Geometry: final body of the model. Coordinates: model frame, mm. A direction names the side the tool comes from. Give positions to 0.01 mm unless a question says otherwise; leave off trailing zeros. Loops run counter-clockwise (first coordinate to the right, second up) from the corner with the lowest first, then second, coordinate; pieces in that order, holes last.
from build123d import *

# Parameters (mm, degrees)
BOSS_EXTRUDE1_DEPTH       = 34.31697226
SKETCH4_R                 = 19.05
BOSS_EXTRUDE2_DEPTH       = 12.7
SKETCH6_R                 = 12.7
BOSS_EXTRUDE3_DEPTH       = 88.9
SKETCH7_R                 = 6.35
CUT_EXTRUDE1_DEPTH        = 141.870111622
FILLET1_R                 = 5.08
FILLET2_R                 = 2.54
M6X1_0_TAPPED_HOLE1_D     = 5
M6X1_0_TAPPED_HOLE1_DEPTH = 41.148
M6X1_0_TAPPED_HOLE1_TIP   = 1.502151548


with BuildPart() as part:
    # Sketch3 → Boss-Extrude1 (new body)
    with BuildSketch(Plane(origin=(0, 0, 0), x_dir=(1, 0, 0), z_dir=(0, 1, 0))):
        Polygon((12.7, 0), (12.7, 12.7), (0, 12.7), (-12.7, 12.7), (-12.7, 0), (-12.7, -12.7), (0, -12.7), (12.7, -12.7), align=None)
    extrude(amount=BOSS_EXTRUDE1_DEPTH)

    # Sketch4 → Boss-Extrude2 (add)
    with BuildSketch(Plane(origin=(0, 34.31697226, 0), x_dir=(1, 0, 0), z_dir=(0, 1, 0))):
        with Locations(Location((0, 0, 0), (0, 0, 270))):
            Circle(SKETCH4_R)
    extrude(amount=BOSS_EXTRUDE2_DEPTH)

    # Sketch6 → Boss-Extrude3 (add)
    with BuildSketch(Plane(origin=(0, 47.01697226, 0), x_dir=(1, 0, 0), z_dir=(0, 1, 0))):
        with Locations(Location((0, 0, 0), (0, 0, 270))):
            Circle(SKETCH6_R)
    extrude(amount=BOSS_EXTRUDE3_DEPTH)

    # Sketch7 → Cut-Extrude1 (cut, through all)
    with BuildSketch(Plane.XY.offset(12.7)):
        with Locations((0, 12.7)):
            Circle(SKETCH7_R)
    extrude(amount=-CUT_EXTRUDE1_DEPTH, mode=Mode.SUBTRACT)

    # Fillet1
    fillet1_edges = [part.edges().sort_by_distance(p)[0] for p in [
        (12.7, 0, 0),
        (-12.7, 0, 0),
    ]]
    fillet(fillet1_edges, radius=FILLET1_R)

    # Fillet2
    fillet2_edges = [part.edges().sort_by_distance(p)[0] for p in [
        (0, 47.01697226, -12.7),
    ]]
    fillet(fillet2_edges, radius=FILLET2_R)

    # M6x1.0 Tapped Hole1
    with Locations(Plane(origin=(0, 135.91697226, 0), x_dir=(1, 0, 0), z_dir=(0, 1, 0))):
        with Locations((0, 0)):
            Hole(M6X1_0_TAPPED_HOLE1_D / 2, depth=M6X1_0_TAPPED_HOLE1_DEPTH)
            with Locations((0, 0, -(M6X1_0_TAPPED_HOLE1_DEPTH + M6X1_0_TAPPED_HOLE1_TIP / 2))):  # 118° drill point
                Cone(0, M6X1_0_TAPPED_HOLE1_D / 2, M6X1_0_TAPPED_HOLE1_TIP, mode=Mode.SUBTRACT)


solid = part.part
Item 1: Pin query (flat end, axial travel): pin 1 (5 mm diameter, centred on y = 53, z = 4.5, fed in from -X); pin 2 (20.5 mm diameter, centred on y = 20.5, z = -4, fed in from -X); pin 3 (3 mm diameter, centred on x = -9.5, z = -14.5, fed in from +Y). Return the tip coordinate at first contact, or that it passes through.
Values follow:
pin 1: stops at x = -12.54
pin 2: stops at x = -12.7
pin 3: stops at y = 47.02
Item 2: Section query D-D on y = 39. Return loops of the section in (x, z).
Values follow:
outline: circle Ø38.1 at (0, 0)
Item 3: Section query A-A on y = 12.7. Return loops of the section in (x, z).
Values follow:
outline: (-12.7, -12.7) - (-6.35, -12.7) - (-6.35, 12.7) - (-12.7, 12.7) - close; (6.35, -12.7) - (12.7, -12.7) - (12.7, 12.7) - (6.35, 12.7) - close
Item 4: Section query C-C on y = 85.5. Return loops of the section in (x, z), plus the area to 3 significant figures.
Values follow:
outline: circle Ø25.4 at (0, 0)
area: 507 mm2
Item 5: Section query B-B on y = 115.5. Return loops of the section in (x, z), plus the area to 3 significant figures.
Values follow:
outline: circle Ø25.4 at (0, 0); hole circle Ø5 at (0, 0)
area: 487 mm2
Item 6: Ray query, probe 1 along Y at (x, z) = (-3.5, -16); probe 2 along Z at (x, y) = (11, 28); probe 3 along Z at (x, y) = (-11, 67.5). Return the intervals inside material, ascending.
Values follow:
probe 1: y = 34.32 to 47.02
probe 2: z = -12.7 to 12.7
probe 3: z = -6.35 to 6.35
Item 7: Set-up query: faces 4 (the face through (0, 21, -12.7)), 5 (the face through (0, 21, 12.7)), 6 (the face through (-12.7, 19, 0)). Return all of +Z, -Z, +X, -X, +Y, -Y with unobstructed straight access to the full face (end or side cutting, diameter ignored); none if empty.
Values follow:
face 4: -Z, +X, -X, -Y
face 5: +Z, +X, -X, -Y
face 6: +Z, -Z, -X, -Y
Item 8: Draft query along Z for faces 1 (the face through (13, 47.017, -9)), 2 (the face through (0.54, 115.05, 2.44)), 3 (the face through (-11.59, 40.58, -15.12)). Return one class per face: +Z half, -Z half, draft (parallel to the pull), parting line (faces both ways), or undercut.
Values follow:
face 1: draft
face 2: undercut
face 3: parting line
